Here's the drawing with two shaded views (mm, measured from the low corner). I have some questions. A direction names the side the tool comes from. Give positions to 0.01 mm unless a question says otherwise; leave off trailing zeros. Order: outer loops, then holes, each group sorted by start corner. A loop starts at its lowest first (then second) coordinate and runs counter-clockwise, first axis right, second up. Notation, with made-up numbers: M 46.25,-20 L 85.25,-20 A20 cw 85.25,17 Z; hole C -9.75,89 d9. An arc over 180 degrees is marked long. One line per question, with ' | ' between items. Start each with the question number.
1) Please list where these lines run through material, in increasing order: line 1 along Z through (x, y) = (13, 10.75); line 2 along X through (y, z) = (0.6, 27) (1 decimal); line 3 along Y through (x, z) = (2.5, 13). Write a range as [from, to].
2) If we section it at D-D, the plane y = 20.5: Please give me the cut outline in (x, z).
3) If we section it at A-A, the plane x = 5: Please give me the cut outline in (y, z), plus the area to 3 significant figures.
4) For the marked faces 4, 5 and 6, which set-ups out of +Z, -Z, +X, -X, +Y, -Y let a thin tool reach every point of the face, with its end or its side?
5) I'm going to push flat-ended pins straight in: pin 1 Ø6 at (x, y) = (8, 10.5) entering from -Z; pin 2 Ø1 at (x, z) = (14.5, 25.5) entering from +Y; pin 3 Ø6 at (x, y) = (15.5, 10.5) entering from +Z; pin 4 Ø1.6 at (y, z) = (21, 15) entering from -X. Where does each tip first touch, or does it pass through?
6) If we section it at B-B, the plane y = 17.25: Please give me the cut outline in (x, z).
7) Thinking about a two-plate mould opening in Z: for the marked faces 1, 2 and 3, which applies, +Z half, -Z half, draft (parallel to the pull), parting line (faces both ways), or undercut?
8) If we section it at C-C, the plane z = 19: Please give me the cut outline in (x, y), plus the area to 3 significant figures.
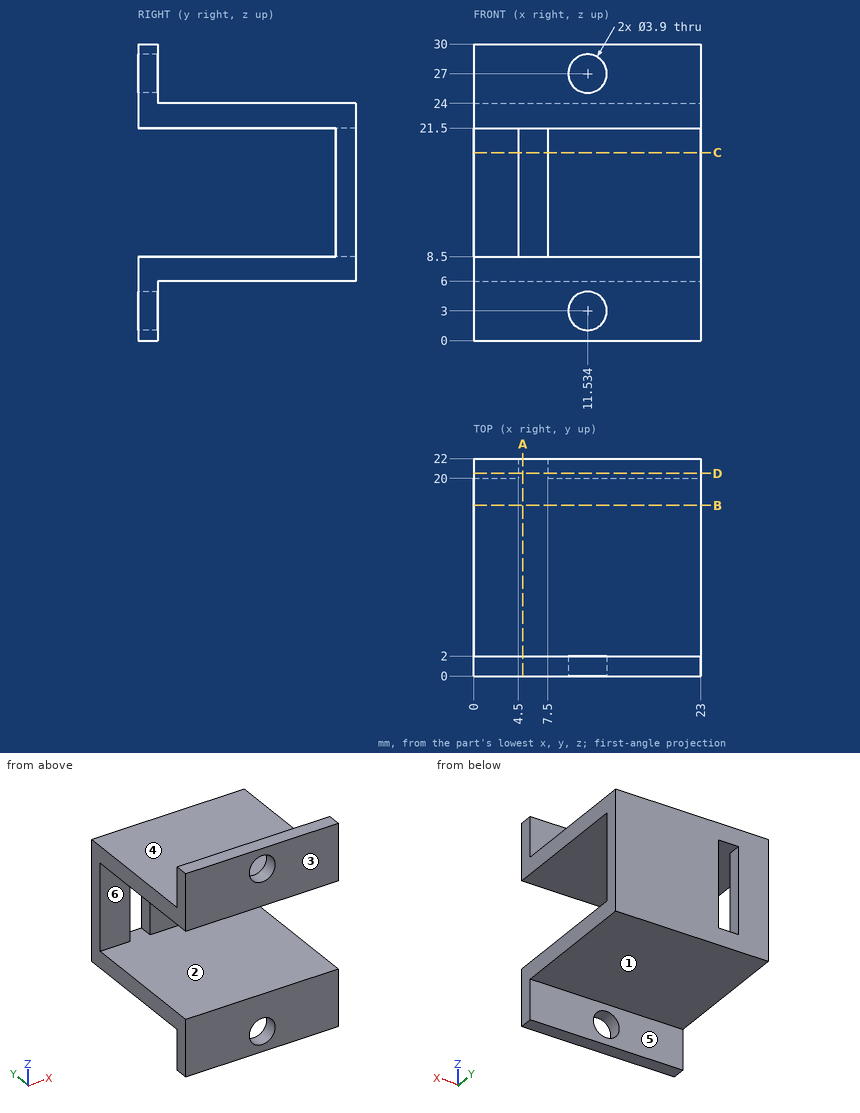
Results found:
1) line 1: z = [6, 8.5], [21.5, 24] | line 2: x = [0, 9.6], [13.5, 23] | line 3: y = [20, 22]
2) outline: M 0,6 L 23,6 L 23,24 L 0,24 Z; hole M 4.5,8.5 L 7.5,8.5 L 7.5,21.5 L 4.5,21.5 Z
3) outline: M 0,0 L 2,0 L 2,6 L 22,6 L 22,8.5 L 0,8.5 Z; M 0,21.5 L 22,21.5 L 22,24 L 2,24 L 2,30 L 0,30 Z | area: 134 mm²
4) face 4: +Z, +X, -X, +Y | face 5: -Z, +X, -X, +Y | face 6: +X, -X, -Y
5) pin 1: stops at z = 6 | pin 2: stops at y = 2 | pin 3: stops at z = 24 | pin 4: stops at x = 0
6) outline: M 0,6 L 23,6 L 23,8.5 L 0,8.5 Z; M 0,21.5 L 23,21.5 L 23,24 L 0,24 Z
7) face 1: -Z half | face 2: undercut | face 3: draft
8) outline: M 0,20 L 4.5,20 L 4.5,22 L 0,22 Z; M 7.5,20 L 23,20 L 23,22 L 7.5,22 Z | area: 40.0 mm²
